Read the model definition and answer for the solid it produces. Units are mm, in the model's axes. Face numbers are marked on the shaded views. A direction names the side the tool comes from. Give positions to 0.01 mm unless a question says otherwise; leave off trailing zeros. Order: outer loops, then holes, each group sorted by start corner. A loop starts at its lowest first (then second) coordinate and runs counter-clockwise, first axis right, second up. Notation, with made-up numbers: (27.5, -31) -> (76.5, -31) arc R15 cw to (76.5, -12) -> close; hole circle Ø5 at (37.25, 12.25). An arc over 180 degrees is marked (long way). Use one line per item in the form item = value.
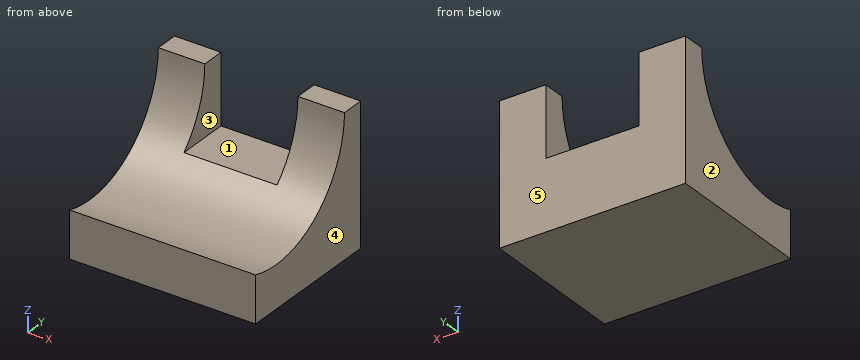
```python
from build123d import *

# Parameters (mm, degrees)
F1_DEPTH = 50.8
F3_DEPTH = 50.8
F4_W     = 25.4
F4_H     = 19.05
F5_DEPTH = 19.05
F6_W     = 25.4
F6_H     = 19.05
F7_DEPTH = 19.05


with BuildPart() as f1:
    # F0 (on Right) → F1 (new body)
    with BuildSketch(Plane.YZ):
        Polygon((54.258809, 18.462197), (54.258809, 56.562197), (47.908809, 56.562197), (13.055639, 31.162197), (13.055639, 18.462197), align=None)
    extrude(amount=F1_DEPTH)

    # F2 (on face) → F3 (cut)
    with BuildSketch(Plane(origin=(0, 0, 0), x_dir=(0, -1, 0), z_dir=(-1, 0, 0))):
        with BuildLine():
            Line((-13.055639, 31.162197), (-47.908809, 56.562197))
            ThreePointArc((-47.908809, 56.562197), (-36.867348, 35.100708), (-13.055639, 31.162197))
        make_face()
    extrude(amount=-F3_DEPTH, mode=Mode.SUBTRACT)

    # F4 (on Front) → F5 (cut)
    with BuildSketch(Plane.XZ):
        with Locations((25.4, 49.807958)):
            Rectangle(F4_W, F4_H)
    extrude(amount=-F5_DEPTH, mode=Mode.SUBTRACT)

    # F6 (on face) → F7 (cut)
    with BuildSketch(Plane(origin=(0, 54.258809, 0), x_dir=(-1, 0, 0), z_dir=(0, 1, 0))):
        with Locations((-25.4, 47.037197)):
            Rectangle(F6_W, F6_H)
    extrude(amount=-F7_DEPTH, mode=Mode.SUBTRACT)


solid = f1.part
```
Item 1: The part is cut by section A-A on x = 42.5. Give the vertices of the cut face in (y, z), and give its area (3 significant figures).
Checks:
outline = (13.06, 18.46) -> (54.26, 18.46) -> (54.26, 56.56) -> (47.91, 56.56) arc R26.87 cw to (13.06, 31.16) -> close
area = 800 mm²
Item 2: Determine the mould class of the marked faces 3, 4 and 5 for opening direction X: +X half, -X half, draft (parallel to the pull), parting line (faces both ways), or undercut.
Checks:
face_3 = undercut
face_4 = +X half
face_5 = draft
Item 3: Which of the six approach directions +Z, -Z, +X, -X, +Y, -Y give full straight-line access (tool end or side, diameter ignored) to the marked faces 1 and 2?
Checks:
face_1 = +Z, +Y, -Y
face_2 = +Z, -Z, -X, +Y, -Y
Item 4: Straight lines are drawn through the part: L1, parallel to X at y = 51.5, z = 43; L2, parallel to Z at x = 22.5, y = 46.5; L3, parallel to Z at x = 10, y = 21. For each, find the intervals that lie inside material, in ascending order. Write a range as from..to.
Checks:
L1 = 0..12.7, 38.1..50.8
L2 = 18.46..37.51
L3 = 18.46..29.95
Item 5: The part is cut by section D-D on z = 47. Give the vertices of the cut face in (x, y), and give its area (3 significant figures).
Checks:
outline = (0, 46.05) -> (12.7, 46.05) -> (12.7, 54.26) -> (0, 54.26) -> close; (38.1, 46.05) -> (50.8, 46.05) -> (50.8, 54.26) -> (38.1, 54.26) -> close
area = 208 mm²
Item 6: The part is cut by section C-C on y = 33. Give the vertices of the cut face in (x, z).
Checks:
outline = (0, 18.46) -> (50.8, 18.46) -> (50.8, 32.75) -> (0, 32.75) -> close
Item 7: Given pin 1 Ø12 at (x, z) = (11, 51) entering from -Y; pin 2 Ø7.5 at (x, y) = (26.5, 47.5) entering from +Z; pin 3 Ø4 at (x, y) = (26.5, 26) entering from +Z, each flat-ended and moving along its own axis, determine where each tip first touches the part or whether it passes through.
Checks:
pin_1 = 45.17
pin_2 = 37.51
pin_3 = 30.86
Item 8: The part is cut by section B-B on z = 54.5. Give the vertices of the cut face in (x, y), and give its area (3 significant figures).
Checks:
outline = (0, 47.81) -> (12.7, 47.81) -> (12.7, 54.26) -> (0, 54.26) -> close; (38.1, 47.81) -> (50.8, 47.81) -> (50.8, 54.26) -> (38.1, 54.26) -> close
area = 164 mm²
